```python
from build123d import *

# Parameters (mm, degrees)
SKETCH_1_W          = 12
SKETCH_1_H          = 16
SKETCH_1_R          = 1.5
EXTRUDE_1_DEPTH     = 8
CUT_EXTRUDE_1_DEPTH = 25
EXTRUDE_2_DEPTH     = 10
FILLET_1_R          = 2
SKETCH_4_R          = 2
CUT_EXTRUDE_2_DEPTH = 20


with BuildPart() as part:
    # 草图1 → 凸台-拉伸1 (new body)
    with BuildSketch(Plane(origin=(0, 0, 0), x_dir=(1, 0, 0), z_dir=(0, 1, 0))):
        Rectangle(SKETCH_1_W, SKETCH_1_H)
        with Locations(Location((2, 5, 0), (0, 0, 270))):
            Circle(SKETCH_1_R, mode=Mode.SUBTRACT)
        with Locations(Location((2, -5, 0), (0, 0, 90))):
            Circle(SKETCH_1_R, mode=Mode.SUBTRACT)
    extrude(amount=EXTRUDE_1_DEPTH)

    # 草图2 → 切除-拉伸1 (cut)
    with BuildSketch(Plane(origin=(6, 0, 0), x_dir=(0, 0, -1), z_dir=(1, 0, 0))):
        with BuildLine():
            Line((-2.039607805, 5.8), (2.039607805, 5.8))
            ThreePointArc((2.039607805, 5.8), (0, 11), (-2.039607805, 5.8))
        make_face()
    extrude(amount=-CUT_EXTRUDE_1_DEPTH, mode=Mode.SUBTRACT)

    # 草图3 → 凸台-拉伸2 (add)
    with BuildSketch(Plane.ZY.offset(6)):
        with BuildLine():
            Line((-8, 8), (-4.5, 8))
            ThreePointArc((-4.5, 8), (0, 3.5), (4.5, 8))
            Line((4.5, 8), (8, 8))
            ThreePointArc((8, 8), (0, 0), (-8, 8))
        make_face()
    extrude(amount=EXTRUDE_2_DEPTH)

    # 圆角1
    # the kernel refuses this fillet: 2 mm, written as the material it takes off along each edge
    with BuildSketch(Plane(origin=(11, 0, 8), x_dir=(0, 0, -1), z_dir=(-1, 0, 0))) as fillet_1_piece_1:
        with BuildLine():
            CenterArc((FILLET_1_R, -FILLET_1_R), FILLET_1_R, 90, 90)
            Line((0, -FILLET_1_R), (0, 0))
            Line((0, 0), (FILLET_1_R, 0))
        make_face()
    extrude(amount=22, mode=Mode.SUBTRACT)
    with BuildSketch(Plane(origin=(-11, 0, -8), x_dir=(0, 1, 0), z_dir=(1, 0, 0))) as fillet_1_piece_2:
        with BuildLine():
            CenterArc((FILLET_1_R, FILLET_1_R), FILLET_1_R, 180, 90)
            Line((0, FILLET_1_R), (0, 0))
            Line((0, 0), (FILLET_1_R, 0))
        make_face()
    extrude(amount=22, mode=Mode.SUBTRACT)

    # 草图4 → 切除-拉伸2 (cut)
    with BuildSketch(Plane(origin=(0, 8, 0), x_dir=(1, 0, 0), z_dir=(0, 1, 0))):
        with Locations(Location((-11, 0, 0), (0, 0, 270))):
            Circle(SKETCH_4_R)
    extrude(amount=-CUT_EXTRUDE_2_DEPTH, mode=Mode.SUBTRACT)


solid = part.part
```
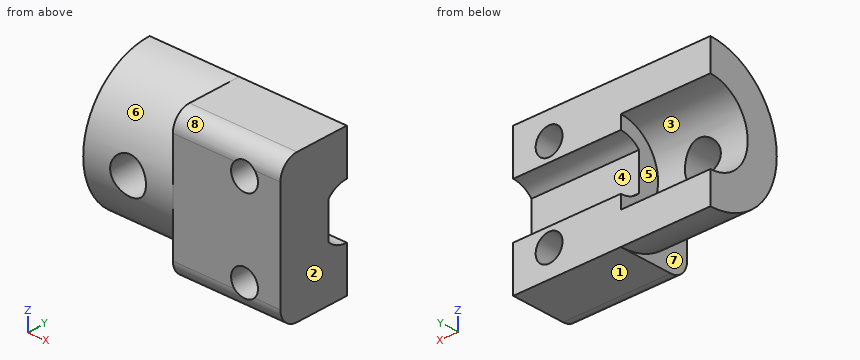
Model file for the job. Use its own axes, mm. Face numbers are marked on the shaded views. A direction names the side the tool comes from. Coordinates: 2 decimals unless noted, no trailing zeros. Write each loop counter-clockwise with the first axis right and the second up, starting at its lowest first coordinate (ties: lowest second). Pieces come first, ordered by that corner, then holes. Notation, with made-up numbers: (12.25, 12.5) - (26.25, 12.5) arc R18 cw to (26.25, 40.5) - close; hole circle Ø9 at (9, -26). An arc over 180 degrees is marked (long way). One line per question, with ' | ' between items. Start each with the question number.
Q1. Drill centre lines: line 1 (X direction, y = 2, z = 5); line 2 (X direction, y = 1.45, z = 0); line 3 (X direction, y = 5.25, z = 3). Where is each one in solid material? Low to high. Write a range as [from, to].
Q2. Cut at A-A, the plane z = -4. List the corners of the cut face in (x, y), then the cut area to 3 significant figures.
Q3. Pin check, flat tips, straight feed: pin 1 (5 mm diameter, centred on x = -11, z = 0, fed in from +Y); pin 2 (4.5 mm diameter, centred on x = 2.5, z = -0.5, fed in from +Y); pin 3 (2 mm diameter, centred on y = 5.5, z = 1, fed in from -X). Stop position of each tip, or through.
Q4. Cut at D-D, the plane x = -11. List the corners of the cut face in (y, z), then the cut area to 3 significant figures.
Q5. Cut at B-B, the plane x = -3.75. List the corners of the cut face in (y, z), then the cut area to 3 significant figures.
Q6. Pull direction Z, two halves, no side cores. Call the marked faces 1, 2 and 3: pulls with the +Z half, pulls with the -Z half, needs draft (parallel to the pull), parting line crosses it, or undercut.
Q7. 3-axis set-ups, long thin cutter, end or side, ignore diameter. For the marked faces 4, 5, 6, 7 and 8: which of +Z, -Z, +X, -X, +Y, -Y reach the whole face in a straight line?
Q8. Cut at C-C, the plane y = 4.5. List the corners of the cut face in (x, z), then the cut area to 3 significant figures.
Answer below:
1) line 1: [-16, 0.5], [3.5, 6] | line 2: [-16, -13], [-9, 6] | line 3: [-6, 6]
2) outline: (-16, 1.07) - (-6, 1.07) - (-6, 0) - (0.88, 0) - (0.88, 8) - (-6, 8) - (-6, 5.94) - (-16, 5.94) - close; (3.12, 0) - (6, 0) - (6, 8) - (3.12, 8) - close | area: 127 mm^2
3) pin 1: y = 4.26 | pin 2: y = 6.8 | pin 3: x = -6
4) outline: (0.25, -2) arc R8 ccw to (8, -8) - (8, -4.5) arc R4.5 cw to (3.97, -2) - close; (0.25, 2) - (3.97, 2) arc R4.5 cw to (8, 4.5) - (8, 8) arc R8 ccw to start | area: 54.4 mm^2
5) outline: (0, -6) arc R2 ccw to (2, -8) - (8, -8) - (8, -3) arc R3 cw to (5.8, -2.04) - (5.8, 2.04) arc R3 cw to (8, 3) - (8, 8) - (2, 8) arc R2 ccw to (0, 6) - close | area: 114 mm^2
6) face 1: pulls with the -Z half | face 2: needs draft | face 3: undercut
7) face 4: +X, -X, +Y | face 5: -X, +Y | face 6: -X, -Y | face 7: -Z, -X, -Y | face 8: +Z, +X, -X, -Y
8) outline: (-16, -7.19) - (-6, -7.19) - (-6, -8) - (6, -8) - (6, 8) - (-6, 8) - (-6, 7.19) - (-16, 7.19) - (-16, 2.83) - (-6, 2.83) - (-6, -2.83) - (-16, -2.83) - close; hole circle Ø3 at (2, -5); hole circle Ø3 at (2, 5) | area: 265 mm^2
